```python
from build123d import *

# Parameters (mm, degrees)
SKETCH2_W          = 2
SKETCH2_H          = 2
CUT_EXTRUDE1_DEPTH = 10


with BuildPart() as part:
    # Sketch1 → Revolve1 (revolve)
    with BuildSketch(Plane.XY, mode=Mode.PRIVATE) as revolve1_sk:
        Polygon((0, 49.555627393), (6.5, 49.555627393), (2.596444265, 45.652071659), (2.596444265, 33.152071659), (0, 31.653013863), align=None)
    revolve(revolve1_sk.sketch.rotate(Axis((0, 49.555627393, 0), (0, -1, 0)), 180), axis=Axis((0, 49.555627393, 0), (0, -1, 0)))

    # Sketch2 → Cut-Extrude1 (cut, symmetric)
    with BuildSketch(Plane.XY):
        with Locations((0, 49.555627393)):
            Rectangle(SKETCH2_W, SKETCH2_H)
    extrude(amount=CUT_EXTRUDE1_DEPTH, both=True, mode=Mode.SUBTRACT)


solid = part.part
```
Model file for the job. Use its own axes, mm. A direction names the side the tool comes from. Round coordinates to 2 decimals unless told otherwise and drop trailing zeros. Order: outer loops, then holes, each group sorted by start corner. A loop starts at its lowest first (then second) coordinate and runs counter-clockwise, first axis right, second up. Notation, with made-up numbers: (10.5, 73) -> (37.5, 73) arc R22 cw to (37.5, 97) -> close; hole circle Ø9 at (43, 0). An arc over 180 degrees is marked (long way). Use one line per item in the form item = value.
Item 1: Tool access for faces 4 (the face through (2.06, 39.31, 1.58)), 5 (the face through (-1, 49, 0)), 6 (the face through (-3, 49.556, 0)): list every direction of +Z, -Z, +X, -X, +Y, -Y with a clear straight run to the whole face (end or side of a thin tool).
Returned:
face_4 = -Y
face_5 = +Z, -Z, +Y
face_6 = +Z, -Z, +X, -X, +Y
Item 2: Cut at A-A, the plane y = 40.75. Write the cut outline in (x, z), and give its area (3 significant figures).
Returned:
outline = circle Ø5.19 at (0, 0)
area = 21.2 mm^2
Item 3: Drill centre lines: line 1 (Y direction, x = -3.5, z = -3.5); line 2 (X direction, y = 47, z = 3); line 3 (Y direction, x = 3.5, z = -0.75). Where is each one in solid material? Low to high.
Returned:
line_1 = 48.01 to 49.56
line_2 = -2.56 to 2.56
line_3 = 46.64 to 49.56
Item 4: Flat gauge pins, fed straight in: pin 1 Ø1.5 at (x, y) = (-0.5, 42.5) entering from +Z; pin 2 Ø1 at (x, y) = (-2, 38) entering from +Z; pin 3 Ø5 at (y, z) = (41.5, 3) entering from +X. Where does each tip first touch, or does it go through?
Returned:
pin_1 = 2.6
pin_2 = 2.12
pin_3 = 2.55
Item 5: Pull direction X, two halves, no side cores. Call faces 1 (the face through (3, 49.556, 0)), 2 (the face through (0.6, 45.84, 2.72)), 3 (the face through (0, 48.556, 0)): released by +X, released by -X, zero draft, split by the parting line, or undercut.
Returned:
face_1 = zero draft
face_2 = split by the parting line
face_3 = undercut
